Could you check a few things on this drawing? It's one solid part, dimensions in mm from its lowest x, y, z. Coordinates: 2 decimals unless noted, no trailing zeros. Loops run counter-clockwise (first coordinate to the right, second up) from the corner with the lowest first, then second, coordinate; pieces in that order, holes last.
1) Imagine slicing it at C-C on z = 1.45. Please give me the cut outline in (x, y).
2) Will these pins go through, and if not, where does the flat tip stop? P1, Ø6, axis at x = 10, y = 13.5, coming from the -Z side; P2, Ø1.5, axis at x = 6, z = 2.5, coming from the -Y side.
3) If I drill on line 1 along Y through (x, z) = (10, 1.3); line 2 along Y through (x, z) = (11.5, 2); line 3 along X through (y, z) = (14, 1.65), over which ranges is the centre line in solid material (lowest first)?
4) Imagine slicing it at A-A on x = 10. Please give me the cut outline in (y, z), plus the area to 3 significant figures.
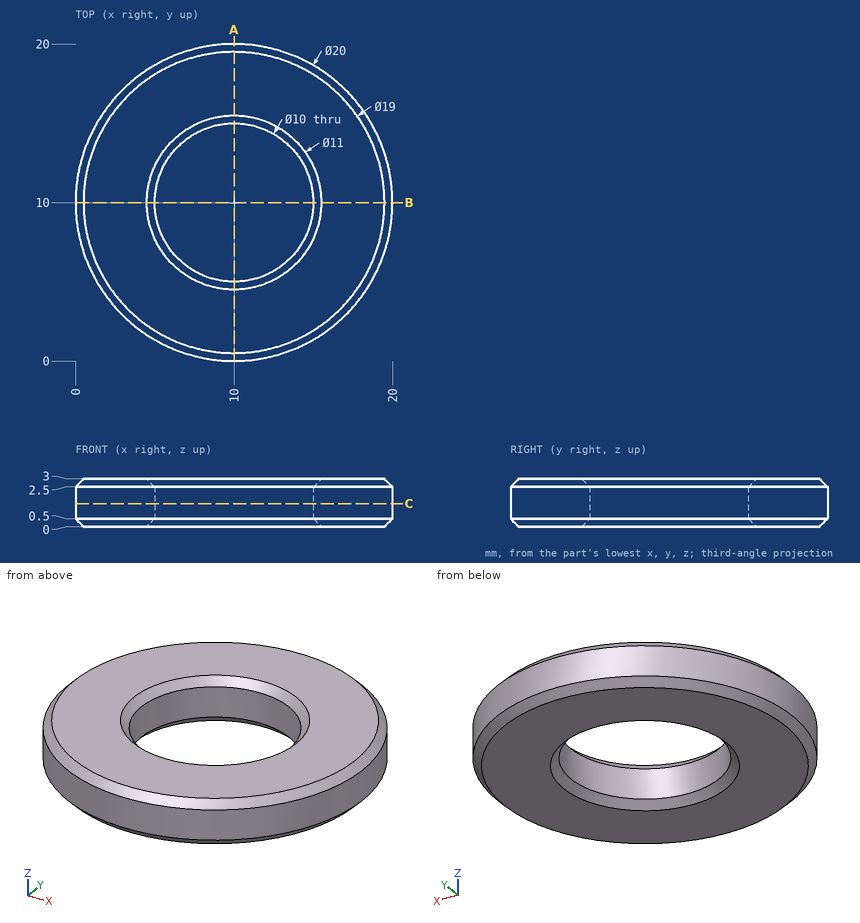
Filled in:
1. outline: circle Ø20 at (10, 10); hole circle Ø10 at (10, 10)
2. P1: stops at z = 0
2. P2: stops at y = 0.54
3. line 1: y = 0 to 5, 15 to 20
3. line 2: y = 0.11 to 5.23, 14.77 to 19.89
3. line 3: x = 0.83 to 7, 13 to 19.17
4. outline: (0, 0.5) - (0.5, 0) - (4.5, 0) - (5, 0.5) - (5, 2.5) - (4.5, 3) - (0.5, 3) - (0, 2.5) - close; (15, 0.5) - (15.5, 0) - (19.5, 0) - (20, 0.5) - (20, 2.5) - (19.5, 3) - (15.5, 3) - (15, 2.5) - close
4. area: 29.0 mm2
